```python
from build123d import *

# Parameters (mm, degrees)
SKETCH1_R           = 350
BOSS_EXTRUDE1_DEPTH = 30
FILLET1_R           = 10
SKETCH2_R           = 4
CUT_EXTRUDE1_DEPTH  = 48


with BuildPart() as part:
    # Sketch1 → Boss-Extrude1 (new body)
    with BuildSketch(Plane(origin=(0, 0, 0), x_dir=(1, 0, 0), z_dir=(0, 1, 0))):
        with Locations(Location((0, 0, 0), (0, 0, 270))):
            Circle(SKETCH1_R)
    extrude(amount=BOSS_EXTRUDE1_DEPTH)

    # Fillet1
    fillet1_edges = [part.edges().sort_by_distance(p)[0] for p in [
        (0, 0, -350),
        (0, 30, -350),
    ]]
    fillet(fillet1_edges, radius=FILLET1_R)

    # Sketch2 → Cut-Extrude1 (cut, symmetric)
    with BuildSketch(Plane(origin=(0, 30, 0), x_dir=(1, 0, 0), z_dir=(0, 1, 0))):
        with Locations(Location((0, 225, 0), (0, 0, 270))):
            Circle(SKETCH2_R)
        with Locations(Location((225, 0, 0), (0, 0, 270))):
            Circle(SKETCH2_R)
        with Locations(Location((0, -225, 0), (0, 0, 270))):
            Circle(SKETCH2_R)
        with Locations(Location((-225, 0, 0), (0, 0, 270))):
            Circle(SKETCH2_R)
    extrude(amount=CUT_EXTRUDE1_DEPTH, both=True, mode=Mode.SUBTRACT)


solid = part.part
```
Input: part model. Units: mm. Frame: model coordinates. Coordinates: 2 decimals unless noted, no trailing zeros. Loops run counter-clockwise (first coordinate to the right, second up) from the corner with the lowest first, then second, coordinate; pieces in that order, holes last. Notation, with made-up numbers: (-20.75, 71) -> (-13.75, 71) arc R26 ccw to (-13.75, 107) -> close; hole circle Ø1 at (86.25, 73.25). An arc over 180 degrees is marked (long way). Use a Markdown table: item, result.
1) Contact query for flat-ended pins moving along their axis: pin 1 (2 mm diameter, centred on x = 141, y = 9, fed in from +Z); pin 2 (10 mm diameter, centred on x = 88, y = 26, fed in from +Z); pin 3 (10 mm diameter, centred on x = -167.5, y = 18.5, fed in from +Z); pin 4 (5 mm diameter, centred on x = 0, z = 225, fed in from +Y). Output: stop coordinate, or through.
Results found:
| item | result |
|---|---|
| pin 1 | stops at z = 320.74 |
| pin 2 | stops at z = 339.34 |
| pin 3 | stops at z = 309.99 |
| pin 4 | passes through |
2) Pull-direction query (Y, two-part tool) for faces 1 (the cylindrical face through (347.022, 14.93, -45.563)), 2 (the flat face through (5, 0, -5)), 3 (the flat face through (5, 30, -5)); classes: released by +Y, released by -Y, zero draft, split by the parting line, or undercut.
Results found:
| item | result |
|---|---|
| face 1 | zero draft |
| face 2 | released by -Y |
| face 3 | released by +Y |
3) Material intervals for line 1 along X through (y, z) = (19.75, 0); line 2 along X through (y, z) = (20.5, 0); line 3 along X through (y, z) = (22, -225), sorted ascending. Write a range as from..to.
Results found:
| item | result |
|---|---|
| line 1 | x = -350..-229, -221..221, 229..350 |
| line 2 | x = -349.99..-229, -221..221, 229..349.99 |
| line 3 | x = -267.83..-4, 4..267.83 |
4) Cut plane A-A (y = 4.75). Return the cut outline in (x, z), then the cut area to 3 significant figures.
Results found:
| item | result |
|---|---|
| outline | circle Ø697.02 at (0, 0); hole circle Ø8 at (-225, 0); hole circle Ø8 at (0, -225); hole circle Ø8 at (0, 225); hole circle Ø8 at (225, 0) |
| area | 381,000 mm2 |
